Input: part model. Units: mm. Frame: model coordinates. Face numbers are marked on the shaded views. A direction names the side the tool comes from. Coordinates: 2 decimals unless noted, no trailing zeros. Write each loop counter-clockwise with the first axis right and the second up, starting at its lowest first coordinate (ties: lowest second). Pieces come first, ordered by that corner, then holes.
1) Draft query along Z for the marked faces 5, 6 and 7. Return one class per face: pulls with the +Z half, pulls with the -Z half, needs draft (parallel to the pull), parting line crosses it, or undercut.
2) Section query D-D (y = -4.5). Output: boundary loops of the cut face in (x, z), then the cut area to 3 significant figures.
3) Section query B-B (z = 14.25). Output: boundary loops of the cut face in (x, y).
4) Pin query (flat end, axial travel): pin 1 Ø2 at (y, z) = (1.5, 4.5) entering from +X; pin 2 Ø8 at (x, z) = (-3, 9.5) entering from +Y; pin 3 Ø1.1 at (x, z) = (0, 9) entering from -Y. Return the tip coordinate at first contact, or that it passes through.
5) Line query: L1, parallel to Z at x = -13.25, y = 3.5; L2, parallel to Y at x = 0, z = 4.25; L3, parallel to Y at x = 0, z = 5.5. Output: solid intervals per line, ascending.
6) Section query A-A (x = 0). Output: boundary loops of the cut face in (y, z).
7) Section query C-C (y = 0). Output: boundary loops of the cut face in (x, z).
8) Set-up query: the marked faces 1, 2, 3 and 4. Return all of +Z, -Z, +X, -X, +Y, -Y with unobstructed straight access to the full face (end or side cutting, diameter ignored); none if empty.
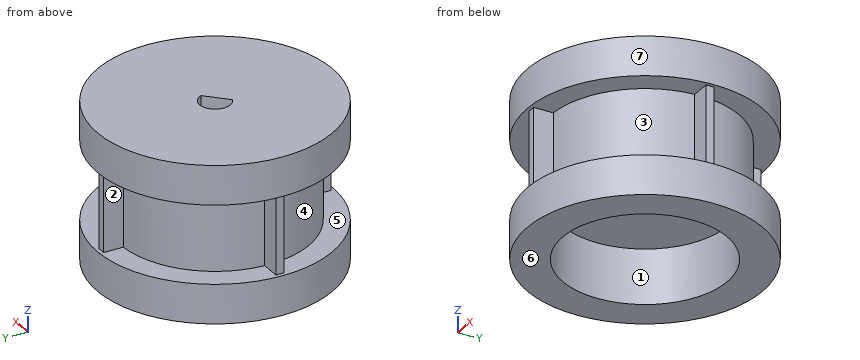
from build123d import *

# Parameters (mm, degrees)
BOX006_W                    = 10
BOX006_H                    = 10
BOX006_DEPTH                = 20
CYLINDER016_R               = 1.95
CYLINDER016_DEPTH           = 20
CUT001_PLACEMENT_ANGLE      = 315
CYLINDER015_R               = 10.5
CYLINDER015_DEPTH           = 7
CYLINDER010_R               = 12
CYLINDER010_DEPTH           = 20
CYLINDER011_R               = 15
CYLINDER011_DEPTH           = 3.5
CYLINDER012_R               = 15
CYLINDER012_DEPTH           = 1.5
CYLINDER013_R               = 15
CYLINDER013_DEPTH           = 1.5
CYLINDER014_R               = 15
CYLINDER014_DEPTH           = 3.5
BOX004_W                    = 29
BOX004_H                    = 1
BOX004_DEPTH                = 10
BOX005_W                    = 29
BOX005_H                    = 1
BOX005_DEPTH                = 10
COMPOUND002_PLACEMENT_ANGLE = 90


with BuildPart() as cube006:
    # Box006 → Box006 (new body)
    with BuildSketch(Plane(origin=(0.75, -5, 0), x_dir=(1, 0, 0), z_dir=(0, 0, 1))):
        with Locations((5, 5)):
            Rectangle(BOX006_W, BOX006_H)
    extrude(amount=BOX006_DEPTH)


with BuildPart() as n20motorshaft:
    # Cylinder016 → Cylinder016 (new body)
    with BuildSketch(Plane.XY):
        Circle(CYLINDER016_R)
    extrude(amount=CYLINDER016_DEPTH)

    # Cut001: cut Cube006
    add(cube006.part, mode=Mode.SUBTRACT)


with BuildPart() as n20motorshaft_1:
    # Cut001 placement: moved
    add(n20motorshaft.part.rotate(Axis((0, 0, 0), (0, 0, 1)), CUT001_PLACEMENT_ANGLE))


with BuildPart() as cylinder015:
    # Cylinder015 → Cylinder015 (new body)
    with BuildSketch(Plane.XY):
        Circle(CYLINDER015_R)
    extrude(amount=CYLINDER015_DEPTH)


with BuildPart() as cylinder010:
    # Cylinder010 → Cylinder010 (new body)
    with BuildSketch(Plane.XY):
        Circle(CYLINDER010_R)
    extrude(amount=CYLINDER010_DEPTH)


with BuildPart() as cylinder011:
    # Cylinder011 → Cylinder011 (new body)
    with BuildSketch(Plane.XY):
        Circle(CYLINDER011_R)
    extrude(amount=CYLINDER011_DEPTH)


with BuildPart() as cylinder012:
    # Cylinder012 → Cylinder012 (new body)
    with BuildSketch(Plane.XY.offset(3.5)):
        Circle(CYLINDER012_R)
    extrude(amount=CYLINDER012_DEPTH)


with BuildPart() as cylinder013:
    # Cylinder013 → Cylinder013 (new body)
    with BuildSketch(Plane.XY.offset(18.5)):
        Circle(CYLINDER013_R)
    extrude(amount=CYLINDER013_DEPTH)


with BuildPart() as cylinder014:
    # Cylinder014 → Cylinder014 (new body)
    with BuildSketch(Plane.XY.offset(15)):
        Circle(CYLINDER014_R)
    extrude(amount=CYLINDER014_DEPTH)


with BuildPart() as cube004:
    # Box004 → Box004 (new body)
    with BuildSketch(Plane(origin=(-14.5, -0.5, 5), x_dir=(1, 0, 0), z_dir=(0, 0, 1))):
        with Locations((14.5, 0.5)):
            Rectangle(BOX004_W, BOX004_H)
    extrude(amount=BOX004_DEPTH)


with BuildPart() as obj1:
    # Box005 → Box005 (new body)
    with BuildSketch(Plane(origin=(-14.5, -0.5, 5), x_dir=(1, 0, 0), z_dir=(0, 0, 1))):
        with Locations((14.5, 0.5)):
            Rectangle(BOX005_W, BOX005_H)
    extrude(amount=BOX005_DEPTH)


with BuildPart() as obj1_1:
    # Compound002 placement: moved
    add(obj1.part.rotate(Axis((0, 0, 0), (0, 0, 1)), COMPOUND002_PLACEMENT_ANGLE))

    # Fusion002: union Cylinder010, Cylinder011, Cylinder012, Cylinder013, Cylinder014, Cube004
    add(cylinder010.part)
    add(cylinder011.part)
    add(cylinder012.part)
    add(cylinder013.part)
    add(cylinder014.part)
    add(cube004.part)

    # Cut: cut Cylinder015
    add(cylinder015.part, mode=Mode.SUBTRACT)

    # Cut002: cut N20MotorShaft
    add(n20motorshaft_1.part, mode=Mode.SUBTRACT)


solid = obj1_1.part
Answer:
1. face 5: undercut
1. face 6: pulls with the -Z half
1. face 7: needs draft
2. outline: (-14.31, 0) - (-9.49, 0) - (-9.49, 7) - (9.49, 7) - (9.49, 0) - (14.31, 0) - (14.31, 5) - (11.12, 5) - (11.12, 15) - (14.31, 15) - (14.31, 20) - (-14.31, 20) - (-14.31, 15) - (-11.12, 15) - (-11.12, 5) - (-14.31, 5) - close
2. area: 376 mm2
3. outline: (-14.5, -0.5) - (-11.99, -0.5) arc R12 ccw to (-0.5, -11.99) - (-0.5, -14.5) - (0.5, -14.5) - (0.5, -11.99) arc R12 ccw to (11.99, -0.5) - (14.5, -0.5) - (14.5, 0.5) - (11.99, 0.5) arc R12 ccw to (0.5, 11.99) - (0.5, 14.5) - (-0.5, 14.5) - (-0.5, 11.99) arc R12 ccw to (-11.99, 0.5) - (-14.5, 0.5) - close; hole (-0.74, -1.8) - (1.8, 0.74) arc R1.95 ccw (long way) to start
4. pin 1: stops at x = 14.99
4. pin 2: stops at y = 14.5
4. pin 3: stops at y = -14.5
5. L1: z = 0 to 5, 15 to 20
5. L2: y = -15 to -10.5, 10.5 to 15
5. L3: y = -14.5 to -10.5, 10.5 to 14.5
6. outline: (-15, 0) - (-10.5, 0) - (-10.5, 7) - (-1.06, 7) - (-1.06, 20) - (-15, 20) - (-15, 15) - (-14.5, 15) - (-14.5, 5) - (-15, 5) - close; (1.95, 7) - (10.5, 7) - (10.5, 0) - (15, 0) - (15, 5) - (14.5, 5) - (14.5, 15) - (15, 15) - (15, 20) - (1.95, 20) - close
7. outline: (-15, 0) - (-10.5, 0) - (-10.5, 7) - (-1.95, 7) - (-1.95, 20) - (-15, 20) - (-15, 15) - (-14.5, 15) - (-14.5, 5) - (-15, 5) - close; (1.06, 7) - (10.5, 7) - (10.5, 0) - (15, 0) - (15, 5) - (14.5, 5) - (14.5, 15) - (15, 15) - (15, 20) - (1.06, 20) - close
8. face 1: -Z
8. face 2: -X, +Y
8. face 3: +X, -Y
8. face 4: -X, -Y
